```python
from build123d import *

# Parameters (mm, degrees)
EXTRUDE_1_DEPTH    = 4
EXTRUDE_2_DEPTH    = 14
HOLE_WIZARD_M3_1_D = 2.5
HOLE_WIZARD_M3_2_D = 2.5


with BuildPart() as part:
    # 草图1 → 凸台-拉伸1 (new body)
    with BuildSketch(Plane(origin=(0, 0, 0), x_dir=(1, 0, 0), z_dir=(0, 1, 0))):
        with BuildLine():
            ThreePointArc((-8.838834765, 13.030441647), (-12.727922061, 12.727922061), (-13.030441647, 8.838834765))
            ThreePointArc((-13.030441647, 8.838834765), (-10.14964129, 0), (-13.030441647, -8.838834765))
            ThreePointArc((-13.030441647, -8.838834765), (-12.727922061, -12.727922061), (-8.838834765, -13.030441647))
            ThreePointArc((-8.838834765, -13.030441647), (0, -10.14964129), (8.838834765, -13.030441647))
            ThreePointArc((8.838834765, -13.030441647), (12.727922061, -12.727922061), (13.030441647, -8.838834765))
            ThreePointArc((13.030441647, -8.838834765), (10.14964129, 0), (13.030441647, 8.838834765))
            ThreePointArc((13.030441647, 8.838834765), (12.727922061, 12.727922061), (8.838834765, 13.030441647))
            ThreePointArc((8.838834765, 13.030441647), (0, 10.14964129), (-8.838834765, 13.030441647))
        make_face()
        with BuildLine():
            Line((-3, -4), (3, -4))
            ThreePointArc((3, -4), (0, 5), (-3, -4))
        make_face(mode=Mode.SUBTRACT)
    extrude(amount=EXTRUDE_1_DEPTH)

    # 草图2 → 凸台-拉伸2 (add)
    with BuildSketch(Plane(origin=(0, 4, 0), x_dir=(1, 0, 0), z_dir=(0, 1, 0))):
        with BuildLine():
            Line((-2.692582404, 7), (2.692582404, 7))
            ThreePointArc((2.692582404, 7), (7.5, 0), (2.692582404, -7))
            Line((2.692582404, -7), (-2.692582404, -7))
            ThreePointArc((-2.692582404, -7), (-7.5, 0), (-2.692582404, 7))
        make_face()
        with BuildLine():
            Line((-3, -4), (3, -4))
            ThreePointArc((3, -4), (0, 5), (-3, -4))
        make_face(mode=Mode.SUBTRACT)
    extrude(amount=EXTRUDE_2_DEPTH)

    # M3 螺纹孔1 (through all)
    with Locations(Plane(origin=(0, 4, 0), x_dir=(1, 0, 0), z_dir=(0, 1, 0))):
        with Locations((-10.606601718, 10.606601718), (10.606601718, 10.606601718), (10.606601718, -10.606601718), (-10.606601718, -10.606601718)):
            Hole(HOLE_WIZARD_M3_1_D / 2)

    # M3 螺纹孔2 (through all)
    with Locations(Plane.XY.offset(7)):
        with Locations((0, 15)):
            Hole(HOLE_WIZARD_M3_2_D / 2)


solid = part.part
```
The model under review builds one solid part; all positions refer to its coordinate system, in mm. A direction names the side the tool comes from. Coordinates: 2 decimals unless noted, no trailing zeros. Loops run counter-clockwise (first coordinate to the right, second up) from the corner with the lowest first, then second, coordinate; pieces in that order, holes last. Notation, with made-up numbers: (-25.5, 9) -> (24.5, 9) arc R19 cw to (24.5, 41) -> close; hole circle Ø8 at (51, -39.75). An arc over 180 degrees is marked (long way). Answer as CSV lines item,"result".
Item 1: Take a section at C-C, the plane y = 15. State the section outline as (x, z) points.
Results below:
outline,"(-3, 4) -> (-1.25, 4) -> (-1.25, 7) -> (-2.69, 7) arc R7.5 ccw to (-2.69, -7) -> (-1.25, -7) -> (-1.25, -4.84) arc R5 cw to start; (1.25, -7) -> (2.69, -7) arc R7.5 ccw to (2.69, 7) -> (1.25, 7) -> (1.25, 4) -> (3, 4) arc R5 cw to (1.25, -4.84) -> close"
Item 2: For L1, parallel to X at y = 12.75, z = 0; L2, parallel to Y at x = 0, z = -6.35; L3, parallel to Y at x = 12, z = 8, list the stretches that pass through material, from the lowest coordinate up.
Results below:
L1,"x = -7.5 to -5, 5 to 7.5"
L2,"y = 0 to 13.75, 16.25 to 18"
L3,"y = 0 to 4"
Item 3: Take a section at D-D, the plane x = -3.75. State the section outline as (y, z) points, and give its area (3 significant figures).
Results below:
outline,"(0, -10.63) -> (4, -10.63) -> (4, -6.5) -> (18, -6.5) -> (18, -3.31) -> (0, -3.31) -> close; (0, 3.31) -> (18, 3.31) -> (18, 6.5) -> (4, 6.5) -> (4, 10.63) -> (0, 10.63) -> close"
area,"148 mm2"
Item 4: Machinability: for faces 1 (the flat face through (0, 9, 4)), 2 (the cylindrical face through (-7.5, 10.9, 0.1)), 3 (the flat face through (0, 11, 7)), 4 (the flat face through (0, 11, -7)), 5 (the cylindrical face through (7.5, 10.9, -0.1)), which of the approach directions +Z, -Z, +X, -X, +Y, -Y give a long, thin tool a straight path to every point of the face, cutting with its end or side? Answer none if there is none.
Results below:
face 1,"+Y, -Y"
face 2,"-X, +Y"
face 3,"+Z, +X, -X, +Y"
face 4,"-Z, +X, -X, +Y"
face 5,"+X, +Y"
Item 5: Take a section at B-B, the plane z = 0. State the section outline as (x, y) points.
Results below:
outline,"(-10.15, 0) -> (-5, 0) -> (-5, 18) -> (-7.5, 18) -> (-7.5, 4) -> (-10.15, 4) -> close; (5, 0) -> (10.15, 0) -> (10.15, 4) -> (7.5, 4) -> (7.5, 18) -> (5, 18) -> close"
Item 6: Draft analysis for pull direction Y (two halves, no side actions). For faces 6 (the cylindrical face through (-1.19, 15.38, -5.93)), 7 (the flat face through (-6, 4, -6)), 8 (the cylindrical face through (-12.77, 1.972, 12.685)), state which applies: +Y half, -Y half, draft (parallel to the pull), parting line (faces both ways), or undercut.
Results below:
face 6,"undercut"
face 7,"+Y half"
face 8,"draft"
Item 7: Take a section at A-A, the plane x = 0. State the section outline as (y, z) points, and give its area (3 significant figures).
Results below:
outline,"(0, -10.15) -> (4, -10.15) -> (4, -7) -> (13.75, -7) -> (13.75, -5) -> (0, -5) -> close; (0, 4) -> (13.75, 4) -> (13.75, 7) -> (4, 7) -> (4, 10.15) -> (0, 10.15) -> close; (16.25, -7) -> (18, -7) -> (18, -5) -> (16.25, -5) -> close; (16.25, 4) -> (18, 4) -> (18, 7) -> (16.25, 7) -> close"
area,"103 mm2"
Item 8: Insertion check: pin 1 (1 mm diameter, centred on x = 5, y = 12, fed in from +Z); pin 2 (2.5 mm diameter, centred on x = -1.5, y = 8, fed in from -Z); pin 3 (2 mm diameter, centred on x = 10.61, z = 10.61, fed in from +Y); pin 4 (3 mm diameter, centred on x = 0, y = 15, fed in from +Z). Each pin has a flat end and moves straight along its axis. Give the tip position at first contact, or say it passes through.
Results below:
pin 1,"stops at z = 6"
pin 2,"stops at z = -7"
pin 3,"passes through"
pin 4,"stops at z = 7"
